from build123d import *

# Parameters (mm, degrees)
SKETCH_1_W                    = 85
SKETCH_1_H                    = 14
HOLE_WIZARD_M24_1_D           = 26
HOLE_WIZARD_M24_1_CBORE_D     = 120
HOLE_WIZARD_M24_1_CBORE_DEPTH = 5
HOLE_WIZARD_M8_1_D            = 10
HOLE_WIZARD_M8_1_CBORE_D      = 16
HOLE_WIZARD_M8_1_CBORE_DEPTH  = 10


with BuildPart() as part:
    # 草图1 → 旋转1 (revolve)
    with BuildSketch(Plane(origin=(0, 0, 0), x_dir=(1, 0, 0), z_dir=(0, 1, 0))):
        with Locations((42.5, -7)):
            Rectangle(SKETCH_1_W, SKETCH_1_H)
    revolve(axis=Axis((0, 0, 0), (0, 0, 1)))

    # M24 六角头螺栓的柱形沉头孔1 (through all)
    with Locations(Plane(origin=(0, 0, 0), x_dir=(-1, 0, 0), z_dir=(0, 0, -1))):
        with Locations((0, 0)):
            CounterBoreHole(HOLE_WIZARD_M24_1_D / 2, HOLE_WIZARD_M24_1_CBORE_D / 2, HOLE_WIZARD_M24_1_CBORE_DEPTH)

    # M8 六角头螺栓的柱形沉头孔1 (through all)
    with Locations(Plane(origin=(0, 0, 0), x_dir=(-1, 0, 0), z_dir=(0, 0, -1))):
        with Locations((36.25, 62.786841774), (-72.5, 0), (36.25, -62.786841774)):
            CounterBoreHole(HOLE_WIZARD_M8_1_D / 2, HOLE_WIZARD_M8_1_CBORE_D / 2, HOLE_WIZARD_M8_1_CBORE_DEPTH)


solid = part.part
Read the model definition and answer for the solid it produces. Units are mm, in the model's axes. A direction names the side the tool comes from. Coordinates: 2 decimals unless noted, no trailing zeros. Order: outer loops, then holes, each group sorted by start corner. A loop starts at its lowest first (then second) coordinate and runs counter-clockwise, first axis right, second up. Notation, with made-up numbers: (-38.75, -38.75) - (12.25, -38.75) arc R10 ccw to (12.25, -27.75) - close; hole circle Ø8 at (25, 11.25). An arc over 180 degrees is marked (long way). Use one line per item in the form item = value.
(1) Given pin 1 Ø13 at (x, y) = (-36.25, 62.79) entering from -Z; pin 2 Ø10 at (x, y) = (-14.5, 46.5) entering from -Z; pin 3 Ø2 at (x, z) = (24, 6.5) entering from -Y; pin 4 Ø9.5 at (x, y) = (-36.25, -62.79) entering from +Z, each flat-ended and moving along its own axis, determine where each tip first touches the part or whether it passes through.
Computed values:
pin_1 = 10
pin_2 = 5
pin_3 = -81.83
pin_4 = through
(2) Section A-A, the plane x = 0 is taken. Give the vertices of the cut face in (y, z).
Computed values:
outline = (-85, 0) - (-60, 0) - (-60, 5) - (-13, 5) - (-13, 14) - (-85, 14) - close; (13, 5) - (60, 5) - (60, 0) - (85, 0) - (85, 14) - (13, 14) - close
(3) Straight lines are drawn through the part: L1, parallel to Y at x = -36.25, z = 4.5; L2, parallel to Y at x = -36.25, z = 11.2; L3, parallel to X at y = -4.5, z = 4.25. For each, find the intervals that lie inside material, in ascending order.
Computed values:
L1 = -76.88 to -70.79, -54.79 to -47.81, 47.81 to 54.79, 70.79 to 76.88
L2 = -76.88 to -67.79, -57.79 to 57.79, 67.79 to 76.88
L3 = -84.88 to -59.83, 59.83 to 65.89, 79.11 to 84.88
(4) Section C-C, the plane x = -36.25 is taken. Give the vertices of the cut face in (y, z), then the cut area to 3 significant figures.
Computed values:
outline = (-76.88, 0) - (-70.79, 0) - (-70.79, 10) - (-67.79, 10) - (-67.79, 14) - (-76.88, 14) - close; (-57.79, 10) - (-54.79, 10) - (-54.79, 0) - (-47.81, 0) - (-47.81, 5) - (47.81, 5) - (47.81, 0) - (54.79, 0) - (54.79, 10) - (57.79, 10) - (57.79, 14) - (-57.79, 14) - close; (67.79, 10) - (70.79, 10) - (70.79, 0) - (76.88, 0) - (76.88, 14) - (67.79, 14) - close
area = 1,270 mm²
(5) For a pull along Y with two mould halves and no side action, classify faces 3 (the face through (-67.453, -51.721, 6.902)), 4 (the face through (1, 14, 5)), 5 (the face through (1, -18, 14)) as pulls with the +Y half, pulls with the -Y half, needs draft (parallel to the pull), parting line crosses it, or undercut.
Computed values:
face_3 = parting line crosses it
face_4 = undercut
face_5 = needs draft
(6) Which of the six approach directions +Z, -Z, +X, -X, +Y, -Y give full straight-line access (tool end or side, diameter ignored) to faces 1 (the face through (-10.316, -7.91, 9.563)), 2 (the face through (78.849, -4.868, 4.93))?
Computed values:
face_1 = +Z, -Z
face_2 = -Z
(7) Section D-D, the plane x = 21.5 is taken. Give the vertices of the cut face in (y, z), then the cut area to 3 significant figures.
Computed values:
outline = (-82.24, 0) - (-56.02, 0) - (-56.02, 5) - (56.02, 5) - (56.02, 0) - (82.24, 0) - (82.24, 14) - (-82.24, 14) - close
area = 1,740 mm²
(8) Section B-B, the plane y = 0 is taken. Give the vertices of the cut face in (x, z), then the cut area to 3 significant figures.
Computed values:
outline = (-85, 0) - (-60, 0) - (-60, 5) - (-13, 5) - (-13, 14) - (-85, 14) - close; (13, 5) - (60, 5) - (60, 0) - (64.5, 0) - (64.5, 10) - (67.5, 10) - (67.5, 14) - (13, 14) - close; (77.5, 10) - (80.5, 10) - (80.5, 0) - (85, 0) - (85, 14) - (77.5, 14) - close
area = 1,350 mm²
